Here's how the part is built. I have some questions about the finished solid (model axes, mm). A direction names the side the tool comes from. Round coordinates to 2 decimals unless told otherwise and drop trailing zeros. Write each loop counter-clockwise with the first axis right and the second up, starting at its lowest first coordinate (ties: lowest second). Pieces come first, ordered by that corner, then holes. Notation, with made-up numbers: (4.25, 66.5) -> (17.25, 66.5) arc R13 ccw to (17.25, 90.5) -> close; hole circle Ø6 at (39, -15.5). An arc over 180 degrees is marked (long way). Answer as CSV lines item,"result".
from build123d import *

# Parameters (mm, degrees)
SKETCH1_R           = 1.25
SKETCH1_R_2         = 3
BOSS_EXTRUDE2_DEPTH = 2
CUT_EXTRUDE2_DEPTH  = 2
BOSS_EXTRUDE3_DEPTH = 2
FILLET1_R           = 1


with BuildPart() as part:
    # Sketch1 → Boss-Extrude2 (new body)
    with BuildSketch(Plane(origin=(0, 0, 0), x_dir=(1, 0, 0), z_dir=(0, 1, 0))):
        with BuildLine():
            Line((967.5, -1675.759156323), (1032.5, -1788.342458815))
            ThreePointArc((1032.5, -1788.342458815), (0, -2065), (-1032.5, -1788.342458815))
            Line((-1032.5, -1788.342458815), (-967.5, -1675.759156323))
            ThreePointArc((-967.5, -1675.759156323), (-512.878726771, -1865.792167318), (-25, -1934.838494552))
            Line((-25, -1934.838494552), (-25, -1915))
            Line((-25, -1915), (25, -1915))
            Line((25, -1915), (25, -1934.838494552))
            ThreePointArc((25, -1934.838494552), (512.878726771, -1865.792167318), (967.5, -1675.759156323))
        make_face()
        with Locations((-17, -1925)):
            Circle(SKETCH1_R, mode=Mode.SUBTRACT)
        with Locations((17, -1925)):
            Circle(SKETCH1_R, mode=Mode.SUBTRACT)
        with Locations((962.839745962, -1687.687359553)):
            Circle(SKETCH1_R, mode=Mode.SUBTRACT)
        with Locations((1019.839745962, -1786.414255585)):
            Circle(SKETCH1_R, mode=Mode.SUBTRACT)
        with Locations((686.598290691, -1939.028567923)):
            Circle(SKETCH1_R_2, mode=Mode.SUBTRACT)
        with Locations((933.81836271, -1832.820849255)):
            Circle(SKETCH1_R_2, mode=Mode.SUBTRACT)
        with Locations((427.630331557, -2012.058970193)):
            Circle(SKETCH1_R_2, mode=Mode.SUBTRACT)
        with Locations((-1019.839745962, -1786.414255585)):
            Circle(SKETCH1_R, mode=Mode.SUBTRACT)
        with Locations((-962.839745962, -1687.687359553)):
            Circle(SKETCH1_R, mode=Mode.SUBTRACT)
        with Locations((161.345498888, -2050.662485634)):
            Circle(SKETCH1_R_2, mode=Mode.SUBTRACT)
        with Locations((882.06566784, -1731.244973312)):
            Circle(SKETCH1_R_2, mode=Mode.SUBTRACT)
        with Locations((648.546659607, -1831.566605481)):
            Circle(SKETCH1_R_2, mode=Mode.SUBTRACT)
        with Locations((403.930838218, -1900.549625223)):
            Circle(SKETCH1_R_2, mode=Mode.SUBTRACT)
        with Locations((152.403648196, -1937.013713946)):
            Circle(SKETCH1_R_2, mode=Mode.SUBTRACT)
        with Locations((-152.403648196, -1937.013713946)):
            Circle(SKETCH1_R_2, mode=Mode.SUBTRACT)
        with Locations((-403.930838218, -1900.549625223)):
            Circle(SKETCH1_R_2, mode=Mode.SUBTRACT)
        with Locations((-648.546659607, -1831.566605481)):
            Circle(SKETCH1_R_2, mode=Mode.SUBTRACT)
        with Locations((-882.06566784, -1731.244973312)):
            Circle(SKETCH1_R_2, mode=Mode.SUBTRACT)
        with Locations((-161.345498888, -2050.662485634)):
            Circle(SKETCH1_R_2, mode=Mode.SUBTRACT)
        with Locations((-427.630331557, -2012.058970193)):
            Circle(SKETCH1_R_2, mode=Mode.SUBTRACT)
        with Locations((-933.81836271, -1832.820849255)):
            Circle(SKETCH1_R_2, mode=Mode.SUBTRACT)
        with Locations((-686.598290691, -1939.028567923)):
            Circle(SKETCH1_R_2, mode=Mode.SUBTRACT)
    extrude(amount=BOSS_EXTRUDE2_DEPTH)

    # Sketch2 → Cut-Extrude2 (cut)
    with BuildSketch(Plane(origin=(0, 2, 0), x_dir=(1, 0, 0), z_dir=(0, 1, 0))):
        with BuildLine():
            Line((992.847509482, -1751.163204556), (1012.002075382, -1752.839011927))
            Line((1012.002075382, -1752.839011927), (987.997924618, -1711.262603211))
            Line((987.997924618, -1711.262603211), (979.871933423, -1728.688847565))
            ThreePointArc((979.871933423, -1728.688847565), (977.197403711, -1731.218117373), (973.516351606, -1731.231168973))
            ThreePointArc((973.516351606, -1731.231168973), (945.994067118, -1763.231147456), (987.468003649, -1755.396139162))
            ThreePointArc((987.468003649, -1755.396139162), (989.319832718, -1752.214780325), (992.847509482, -1751.163204556))
        make_face()
    extrude(amount=-CUT_EXTRUDE2_DEPTH, mode=Mode.SUBTRACT)

    # Sketch4 → Boss-Extrude3 (add)
    with BuildSketch(Plane(origin=(0, 2, 0), x_dir=(1, 0, 0), z_dir=(0, 1, 0))):
        with BuildLine():
            Line((-1007.152490518, -1712.938410582), (-987.997924618, -1711.262603211))
            Line((-987.997924618, -1711.262603211), (-1012.002075382, -1752.839011927))
            Line((-1012.002075382, -1752.839011927), (-1020.128066577, -1735.412767573))
            ThreePointArc((-1020.128066577, -1735.412767573), (-1022.802596289, -1732.883497764), (-1026.483648394, -1732.870446165))
            ThreePointArc((-1026.483648394, -1732.870446165), (-1054.005932882, -1700.870467681), (-1012.531996351, -1708.705475976))
            ThreePointArc((-1012.531996351, -1708.705475976), (-1010.680167282, -1711.886834812), (-1007.152490518, -1712.938410582))
        make_face()
        with BuildLine():
            Line((5.48633271, -1906.815018385), (7.679491924, -1915))
            Line((7.679491924, -1915), (-7.679491924, -1915))
            Line((-7.679491924, -1915), (-5.48633271, -1906.815018385))
            ThreePointArc((-5.48633271, -1906.815018385), (-5.549842721, -1905.31863757), (-6.457260037, -1904.127091147))
            ThreePointArc((-6.457260037, -1904.127091147), (0, -1883.819660113), (6.457260037, -1904.127091147))
            ThreePointArc((6.457260037, -1904.127091147), (5.549842721, -1905.31863757), (5.48633271, -1906.815018385))
        make_face()
    extrude(amount=-BOSS_EXTRUDE3_DEPTH)

    # Fillet1
    fillet1_edges = [part.edges().sort_by_distance(p)[0] for p in [
        (-1032.5, 1, 1788.342458815),
        (-967.5, 1, 1675.759156323),
        (-25, 1, 1915),
        (25, 1, 1915),
        (967.5, 1, 1675.759156323),
        (1032.5, 1, 1788.342458815),
    ]]
    fillet(fillet1_edges, radius=FILLET1_R)


solid = part.part
Item 1: Suppose I cut it at B-B, the plane y = 1.65. State how many separate pieces and enclosed holes the cut face has, then the cut area to 3 significant figures.
Results found:
separate pieces,"1"
enclosed holes,"22"
area,"273,000 mm²"
Item 2: Suppose I cut it at C-C, the plane x = -707. List the corners of the cut face in (y, z) for me.
Results found:
outline,"(0, 1801.22) -> (2, 1801.22) -> (2, 1940.2) -> (0, 1940.2) -> close"
Item 3: If we mould it in two halves opening along Z, with no side actions, what happens to faces 1 (the cylindrical face through (-519.06, 0.99, 1864.08)), 2 (the cylindrical face through (945.62, 1.01, 1762.56)), 3 (the flat face through (-8, 0, 1927))? For each: pulls with the +Z half, pulls with the -Z half, needs draft (parallel to the pull), parting line crosses it, or undercut.
Results found:
face 1,"pulls with the -Z half"
face 2,"undercut"
face 3,"needs draft"
Item 4: For faces 4 (the flat face through (-8, 2, 1927)), 5 (the cylindrical face through (505.73, 0.986, 1867.742)), which set-ups out of +Z, -Z, +X, -X, +Y, -Y let a thin tool reach every point of the face, with its end or its side?
Results found:
face 4,"+Z, -Z, +X, -X, +Y"
face 5,"-Z, +Y, -Y"
Item 5: Suppose I cut it at A-A, the plane x = 477.5. List the corners of the cut face in (y, z) for me, then the cut area to 3 significant figures.
Results found:
outline,"(0, 1875.16) -> (2, 1875.16) -> (2, 2009.03) -> (0, 2009.03) -> close"
area,"268 mm²"
Item 6: I need wall thicknesses on L1, parallel to X at y = 0.55, z = 1768; L2, parallel to X at y = 0.7, z = 1710; L3, parallel to Z at x = 153, y = 0.25. Which ranges of each line are inside material? Lowest first, please.
Results found:
L1,"x = -1020.76 to -786.38, 786.38 to 949.69, 981.03 to 1020.76"
L2,"x = -1056.91 to -1012.15, -987.27 to -905.61, 905.61 to 987.27"
L3,"z = 1928.94 to 1934.07, 1939.95 to 2059.32"
Item 7: Will this pin go through, and if not, where does the flat tip stop? pin 1 (3 mm diameter, centred on x = -1019.84, z = 1786.41, fed in from -Y).
Results found:
pin 1,"stops at y = 0"
